Autodesk Inventor part; units mm, degrees
ref_plane "YZ Plane" through (0, 0, 0) normal (1, 0, 0) x (0, 1, 0)
ref_plane "XZ Plane" through (0, 0, 0) normal (0, 1, 0) x (-1, 0, 0)
ref_plane "XY Plane" through (0, 0, 0) normal (0, 0, 1) x (1, 0, 0)
sketch "Sketch1" plane through (0, 0, 0) normal (0, 0, 1) x (1, 0, 0)
  line L0 (-26.5, -5) -> (8.5, -5)
  arc A0 (8.5, -5) -> (8.5, 0) centre (8.5, -2.5) ccw
  line L1 (8.5, 0) -> (0, 0)
  arc A1 (-26.5, -1) -> (-26.5, -5) centre (-26.5, -3) ccw
  line L2 (-26.5, -1) -> (-24.63, -1)
  line L3 (-24.117, -1.0905) -> (-18.8919, -2.9922)
  arc A2 (-24.117, -1.0905) -> (-24.63, -1) centre (-24.63, -2.5) ccw
  line L4 (-18.8919, -2.9922) -> (-19.1314, -3.65) construction
  dimension "d0" = 35
  dimension "d1" = 2.5
  dimension "d2" = 8.5
  dimension "d3" = 1.5
  dimension "d5" = 20
  dimension "d6" = 1.87
  dimension "d7" = 2
  dimension "d8" = 0.7
  dimension "d9" = 1.35
sketch "Sketch2" plane through (0, 0, 0) normal (1, 0, 0) x (0, 1, 0)
  line L0 (0, 0) -> (-0.7, 0)
  line L1 (-0.7, 0) -> (-0.7, 4.5)
  line L2 (-0.7, 4.5) -> (0, 4.5)
  line L3 (0, 4.5) -> (0, 0)
  dimension "d10" = 0.7
  dimension "d11" = 4.5
sweep "Sweep1" add profiles "Sketch2" path "Sketch1"
properties part number "PP-13" material "Steel"
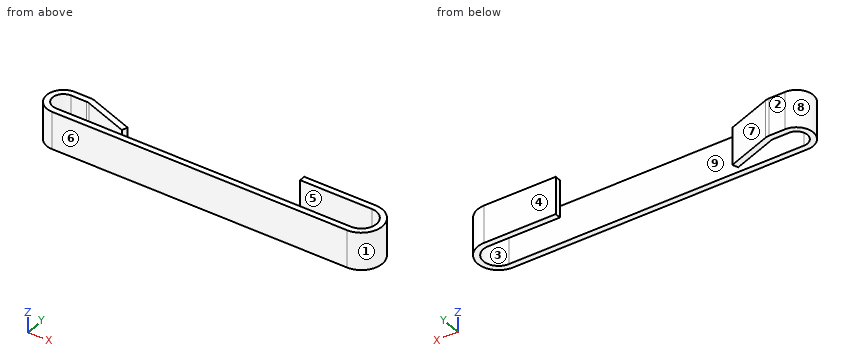
For this review, take the finished solid that the model builds, in its own axes (mm). Face numbers are marked on the shaded views. A direction names the side the tool comes from. Round coordinates to 2 decimals unless told otherwise and drop trailing zeros. Write each loop counter-clockwise with the first axis right and the second up, starting at its lowest first coordinate (ties: lowest second). Pieces come first, ordered by that corner, then holes. Notation, with made-up numbers: (23.5, -27) -> (68.5, -27) arc R27 cw to (68.5, -9) -> close; hole circle Ø10 at (-2.75, -28). An arc over 180 degrees is marked (long way). One line per question, with ' | ' between items. Start each with the question number.
1) Wall thickness on line 1 along Y through (x, z) = (1.5, 4.1); line 2 along Y through (x, z) = (-8, 2.85); line 3 along Y through (x, z) = (-21, 2.25): over which ranges is each line inside the solid? List them lowest first.
2) Add section A-A (x = 2). Write out the cut boundary in (y, z).
3) Add section B-B (z = 1.7). Write out the cut boundary in (x, y).
4) Machinability: for the marked faces 1, 2, 3, 4 and 5, which of the approach directions +Z, -Z, +X, -X, +Y, -Y give a long, thin tool a straight path to every point of the face, cutting with its end or side? Answer none if there is none.
5) Add section D-D (x = -23). Write out the cut boundary in (y, z), and give its area (3 significant figures).
6) For pin 1 Ø0.6 at (y, z) = (0, 2.5) entering from -X; pin 2 Ø1.5 at (x, y) = (0.5, -2.5) entering from -Z; pin 3 Ø1.5 at (x, z) = (-25.5, 3) entering from +Y, all flat-tipped, find the tip position at first contact; note any pin that passes through.
7) Mouldability with a two-part tool opening along Y and no side actions: class the marked faces 6, 7, 8 and 9 as +Y half, -Y half, draft (parallel to the pull), parting line (faces both ways), or undercut.
8) Add section C-C (y = -2.5). Write out the cut boundary in (x, z).
Reported:
1) line 1: y = -5 to -4.3, -0.7 to 0 | line 2: y = -5 to -4.3 | line 3: y = -5 to -4.3, -2.97 to -2.22
2) outline: (-5, 0) -> (-4.3, 0) -> (-4.3, 4.5) -> (-5, 4.5) -> close; (-0.7, 0) -> (0, 0) -> (0, 4.5) -> (-0.7, 4.5) -> close
3) outline: (-26.5, -5) -> (8.5, -5) arc R2.5 ccw to (8.5, 0) -> (0, 0) -> (0, -0.7) -> (8.5, -0.7) arc R1.8 cw to (8.5, -4.3) -> (-26.5, -4.3) arc R1.3 cw to (-26.5, -1.7) -> (-24.63, -1.7) arc R0.8 cw to (-24.36, -1.75) -> (-19.13, -3.65) -> (-18.89, -2.99) -> (-24.12, -1.09) arc R1.5 ccw to (-24.63, -1) -> (-26.5, -1) arc R2 ccw to start
4) face 1: +Z, -Z, +X | face 2: +Z, -Z, -X, +Y | face 3: +Z, -Z | face 4: +Z, -Z, +X, -X, +Y | face 5: +Z, -Z, -X
5) outline: (-5, 0) -> (-4.3, 0) -> (-4.3, 4.5) -> (-5, 4.5) -> close; (-2.24, 0) -> (-1.5, 0) -> (-1.5, 4.5) -> (-2.24, 4.5) -> close | area: 6.50 mm²
6) pin 1: stops at x = 0 | pin 2: passes through | pin 3: stops at y = -1
7) face 6: -Y half | face 7: +Y half | face 8: parting line | face 9: undercut
8) outline: (-28.44, 0) -> (-27.7, 0) -> (-27.7, 4.5) -> (-28.44, 4.5) -> close; (-22.29, 0) -> (-20.24, 0) -> (-20.24, 4.5) -> (-22.29, 4.5) -> close; (10.3, 0) -> (11, 0) -> (11, 4.5) -> (10.3, 4.5) -> close
